from build123d import *

# Parameters (mm, degrees)
SKETCH_1_R             = 36
SKETCH_1_R_2           = 25
EXTRUDE_1_DEPTH        = 10
HOLE_WIZARD_M5_1_D     = 4.2
HOLE_WIZARD_M5_1_DEPTH = 12.4
HOLE_WIZARD_M5_1_TIP   = 1.2618073
MM_1_D                 = 7
MM_1_DEPTH             = 12.4
MM_1_TIP               = 2.103012167


with BuildPart() as part:
    # 草图1 → 凸台-拉伸1 (new body)
    with BuildSketch(Plane.XY):
        Polygon((-11, 90), (56, 90), (56, -90), (-56, -90), (-56, 6), (-11, 6), align=None)
        with Locations((0, -40)):
            Circle(SKETCH_1_R, mode=Mode.SUBTRACT)
        with Locations((22.5, 50)):
            Circle(SKETCH_1_R_2, mode=Mode.SUBTRACT)
    extrude(amount=EXTRUDE_1_DEPTH)

    # M5 螺纹孔1
    with Locations(Plane(origin=(49, -9, 0), x_dir=(-1, 0, 0), z_dir=(0, 0, -1))):
        with Locations((0, 0), (98, 0), (98, -62), (0, -62)):
            Hole(HOLE_WIZARD_M5_1_D / 2, depth=HOLE_WIZARD_M5_1_DEPTH)
            with Locations((0, 0, -(HOLE_WIZARD_M5_1_DEPTH + HOLE_WIZARD_M5_1_TIP / 2))):  # 118° drill point
                Cone(0, HOLE_WIZARD_M5_1_D / 2, HOLE_WIZARD_M5_1_TIP, mode=Mode.SUBTRACT)

    # 大小mm 暗销槽口1
    with Locations(Plane(origin=(47.5, 25, 0), x_dir=(-1, 0, 0), z_dir=(0, 0, -1))):
        with Locations((0, 0), (0, 50), (50, 50), (50, 0)):
            Hole(MM_1_D / 2, depth=MM_1_DEPTH)
            with Locations((0, 0, -(MM_1_DEPTH + MM_1_TIP / 2))):  # 118° drill point
                Cone(0, MM_1_D / 2, MM_1_TIP, mode=Mode.SUBTRACT)


solid = part.part
Could you check a few things on this model? Use its own coordinates, in mm. A direction names the side the tool comes from. Give positions to 0.01 mm unless a question says otherwise; leave off trailing zeros. Order: outer loops, then holes, each group sorted by start corner. A loop starts at its lowest first (then second) coordinate and runs counter-clockwise, first axis right, second up.
1. Suppose I cut it at A-A (z = 5.75). Give the number of separate pieces and of enclosed holes in the cut face, plus the area to 3 significant figures.
2. For faces 1 (the cylindrical face through (-2.96, 28.47, 5.07)), 2 (the flat face through (-34, 6, 5)), which set-ups out of +Z, -Z, +X, -X, +Y, -Y let a thin tool reach every point of the face, with its end or its side?
3. Suppose I cut it at B-B (x = 12.5). List the corners of the cut face in (y, z) for me, plus the area to 3 significant figures.
4. Suppose I cut it at D-D (y = -9). List the corners of the cut face in (x, z) for me.
5. Suppose I cut it at C-C (y = 69.5). List the corners of the cut face in (x, z) for me, plus the area to 3 significant figures.
6. Will these pins go through, and if not, where does the flat tip stop? P1, Ø6, axis at y = 63.5, z = 6.5, coming from the -X side; P2, Ø4, axis at x = -29.5, z = 5.5, coming from the +Y side.
7. I need wall thicknesses on L1, parallel to Y at x = -49, z = 7.5; L2, parallel to Y at x = 31, z = 6.5; L3, parallel to Y at x = 49, z = 8.25. Which ranges of each line are inside material? Lowest first, please.
8. We'd pull the mould along X, two halves only. Please class faces 3 (the flat face through (13, 1, 0)), 4 (the flat face through (-11, 47, 5)), 5 (the cylindrical face through (50.13, -7.23, 5.07)): pulls with the +X half, pulls with the -X half, needs draft (parallel to the pull), parting line crosses it, or undercut.
Solved:
1. separate pieces: 1
1. enclosed holes: 10
1. area: 10,100 mm2
2. face 1: +Z, -Z
2. face 2: +Z, -Z, -X, +Y
3. outline: (-90, 0) - (-73.76, 0) - (-73.76, 10) - (-90, 10) - close; (-6.24, 0) - (27.09, 0) - (27.09, 10) - (-6.24, 10) - close; (72.91, 0) - (90, 0) - (90, 10) - (72.91, 10) - close
3. area: 667 mm2
4. outline: (-56, 0) - (-51.1, 0) - (-51.1, 10) - (-56, 10) - close; (-46.9, 0) - (-18.3, 0) - (-18.3, 10) - (-46.9, 10) - close; (18.3, 0) - (46.9, 0) - (46.9, 10) - (18.3, 10) - close; (51.1, 0) - (56, 0) - (56, 10) - (51.1, 10) - close
5. outline: (-11, 0) - (6.86, 0) - (6.86, 10) - (-11, 10) - close; (38.14, 0) - (56, 0) - (56, 10) - (38.14, 10) - close
5. area: 357 mm2
6. P1: stops at x = -11
6. P2: stops at y = 6
7. L1: y = -90 to -73.1, -68.9 to -11.1, -6.9 to 6
7. L2: y = -90 to -58.3, -21.7 to 26.49, 73.51 to 90
7. L3: y = -90 to -73.1, -68.9 to -11.1, -6.9 to 21.84, 28.16 to 71.84, 78.16 to 90
8. face 3: needs draft
8. face 4: pulls with the -X half
8. face 5: undercut
